```python
from build123d import *

# Parameters (mm, degrees)
CUT_EXTRUDE_1_DEPTH      = 57.291651246
CUT_EXTRUDE_1_DEPTH_BACK = 57.291651246
SKETCH_2_OUTSIDE_W       = 89.516
SKETCH_2_OUTSIDE_H       = 89.516
SKETCH_2_OUTSIDE_W_2     = 16
SKETCH_2_OUTSIDE_H_2     = 65
SKETCH_3_R               = 26
CUT_EXTRUDE_2_DEPTH      = 4
CUT_EXTRUDE_START        = -4
SKETCH_4_R               = 26
CUT_EXTRUDE_3_DEPTH      = 4
SKETCH_5_R               = 5
EXTRUDE_2_DEPTH          = 8
SKETCH_6_R               = 4.25
CUT_EXTRUDE_6_DEPTH      = 4
SKETCH_7_R               = 1.75
CUT_EXTRUDE_7_DEPTH      = 48.502631506


with BuildPart() as part:
    # 草图1 → 旋转3 (revolve)
    with BuildSketch(Plane.XY):
        with BuildLine():
            Line((3.869127368, 32.268868177), (-3.869127368, -32.268868177))
            ThreePointArc((-3.869127368, -32.268868177), (-32.268868177, 3.869127368), (3.869127368, 32.268868177))
        make_face()
    revolve(axis=Axis((3.869127368, 32.268868177, 0), (-0.11905007287477921, -0.9928882515915424, 0)))

    # 草图2 outside → 切除-拉伸1 (cut, two sides: drawn at the far end of the back side and taken through both)
    with BuildSketch(Plane(origin=(0, 0, 0), x_dir=(1, 0, 0), z_dir=(0, 1, 0)).offset(-CUT_EXTRUDE_1_DEPTH_BACK)):
        Rectangle(SKETCH_2_OUTSIDE_W, SKETCH_2_OUTSIDE_H)
        Rectangle(SKETCH_2_OUTSIDE_W_2, SKETCH_2_OUTSIDE_H_2, mode=Mode.SUBTRACT)
    extrude(amount=CUT_EXTRUDE_1_DEPTH + CUT_EXTRUDE_1_DEPTH_BACK, mode=Mode.SUBTRACT)

    # 草图3 → 切除-拉伸2 (cut)
    with BuildSketch(Plane(origin=(8, 0, 0), x_dir=(0, 0, -1), z_dir=(1, 0, 0))):
        Circle(SKETCH_3_R)
    extrude(amount=-CUT_EXTRUDE_2_DEPTH, mode=Mode.SUBTRACT)

    # 草图4 → 切除-拉伸3 (cut)
    with BuildSketch(Plane.ZY.offset(8).offset(CUT_EXTRUDE_START)):
        with Locations(Location((0, 0, 0), (0, 0, 180))):
            Circle(SKETCH_4_R)
    extrude(amount=CUT_EXTRUDE_3_DEPTH, mode=Mode.SUBTRACT)

    # 草图5 → 凸台-拉伸2 (add)
    with BuildSketch(Plane(origin=(4, 0, 0), x_dir=(0, 0, -1), z_dir=(1, 0, 0))):
        Circle(SKETCH_5_R)
        with BuildLine():
            Line((-1.785357107, 1.75), (1.785357107, 1.75))
            ThreePointArc((1.785357107, 1.75), (2.5, 0), (1.785357107, -1.75))
            Line((1.785357107, -1.75), (-1.785357107, -1.75))
            ThreePointArc((-1.785357107, -1.75), (-2.5, 0), (-1.785357107, 1.75))
        make_face(mode=Mode.SUBTRACT)
    extrude(amount=EXTRUDE_2_DEPTH)

    # 草图6 → 切除-拉伸6 (cut)
    with BuildSketch(Plane.ZY.offset(8).offset(CUT_EXTRUDE_START)):
        Circle(SKETCH_6_R)
    extrude(amount=-CUT_EXTRUDE_6_DEPTH, mode=Mode.SUBTRACT)

    # 草图7 → 切除-拉伸7 (cut, through all)
    with BuildSketch(Plane.ZY):
        Circle(SKETCH_7_R)
    extrude(amount=-CUT_EXTRUDE_7_DEPTH, mode=Mode.SUBTRACT)


solid = part.part
```
Input: part model. Units: mm. Frame: model coordinates. A direction names the side the tool comes from. Round coordinates to 2 decimals unless told otherwise and drop trailing zeros. Order: outer loops, then holes, each group sorted by start corner. A loop starts at its lowest first (then second) coordinate and runs counter-clockwise, first axis right, second up. Notation, with made-up numbers: (38.5, -31.75) - (77.5, -31.75) arc R18 ccw to (77.5, -25.75) - close; hole circle Ø9 at (64, 67.25). An arc over 180 degrees is marked (long way). Answer in a Markdown table with one row per item.
Item 1: Mould query, pull axis Z, two halves, no side actions, for faces 1 (the flat face through (-8, -26, -5)), 2 (the cylindrical face through (7.9, 0, -2.5)). Classes: released by +Z, released by -Z, zero draft, split by the parting line, or undercut.
Model answer:
| item | result |
|---|---|
| face 1 | zero draft |
| face 2 | undercut |
Item 2: Line query: line 1 (X direction, y = 4, z = -27); line 2 (Z direction, x = 1.1, y = 0); line 3 (Y direction, x = 7.5, z = 19). Output: solid intervals per line, ascending.
Model answer:
| item | result |
|---|---|
| line 1 | x = -8 to 8 |
| line 2 | z = -32.48 to -1.75, 1.75 to 32.48 |
| line 3 | y = -25.28 to -17.75, 17.75 to 25.28 |
Item 3: Section query B-B (y = 0). Return the cut outline in (x, z).
Model answer:
| item | result |
|---|---|
| outline | (-8, -31.5) arc R32.5 ccw to (8, -31.5) - (8, -26) - (4, -26) - (4, -5) - (12, -5) - (12, -2.5) - (4, -2.5) - (4, -1.75) - (0, -1.75) - (0, -4.25) - (-4, -4.25) - (-4, -26) - (-8, -26) - close; (-8, 26) - (-4, 26) - (-4, 4.25) - (0, 4.25) - (0, 1.75) - (4, 1.75) - (4, 2.5) - (12, 2.5) - (12, 5) - (4, 5) - (4, 26) - (8, 26) - (8, 31.5) arc R32.5 ccw to (-8, 31.5) - close |
Item 4: Section query C-C (z = 15). Return the cut outline in (x, y), then the cut area to 3 significant figures.
Model answer:
| item | result |
|---|---|
| outline | (-8, -27.7) arc R28.83 ccw to (8, -27.7) - (8, -21.24) - (4, -21.24) - (4, 21.24) - (8, 21.24) - (8, 27.7) arc R28.83 ccw to (-8, 27.7) - (-8, 21.24) - (-4, 21.24) - (-4, -21.24) - (-8, -21.24) - close |
| area | 571 mm² |
Item 5: Pin query (flat end, axial travel): pin 1 (3 mm diameter, centred on x = 8.5, z = -0.5, fed in from -Y); pin 2 (1.5 mm diameter, centred on x = 1, y = -25, fed in from -Z); pin 3 (5 mm diameter, centred on x = 9, z = 0, fed in from +Y). Return the tip coordinate at first contact, or that it passes through.
Model answer:
| item | result |
|---|---|
| pin 1 | stops at y = -31.73 |
| pin 2 | stops at z = -21.62 |
| pin 3 | stops at y = 31.84 |
Item 6: Section query D-D (y = 17). Return the cut outline in (x, z), then the cut area to 3 significant figures.
Model answer:
| item | result |
|---|---|
| outline | (-8, -26.52) arc R27.7 ccw to (8, -26.52) - (8, -19.67) - (4, -19.67) - (4, 19.67) - (8, 19.67) - (8, 26.52) arc R27.7 ccw to (-8, 26.52) - (-8, 19.67) - (-4, 19.67) - (-4, -19.67) - (-8, -19.67) - close |
| area | 559 mm² |
Item 7: Reachability of faces 3 (the cylindrical face through (-2.028, 3.584, 2.285)), 4 (the cylindrical face through (7.94, -4.88, 1.08)), 5 (the cylindrical face through (1.972, -0.67, 1.617)) from +Z, -Z, +X, -X, +Y, -Y: full face, straight path, thin tool, end or side. Return the list, or none.
Model answer:
| item | result |
|---|---|
| face 3 | -X |
| face 4 | +X |
| face 5 | +X, -X |
Item 8: Section query A-A (x = 6.5). Return the cut outline in (y, z).
Model answer:
| item | result |
|---|---|
| outline | circle Ø63.69 at (0, 0); circle Ø10 at (0, 0); hole circle Ø52 at (0, 0); hole (-1.75, -1.79) arc R2.5 ccw to (1.75, -1.79) - (1.75, 1.79) arc R2.5 ccw to (-1.75, 1.79) - close |
